```python
from build123d import *

# Parameters (mm, degrees)
SKETCH_1_R          = 16.5
EXTRUDE_1_DEPTH     = 22
SKETCH_2_R          = 18.5
EXTRUDE_2_DEPTH     = 22
SKETCH_3_R          = 6
EXTRUDE_3_DEPTH     = 6
SKETCH_4_R          = 3
EXTRUDE_7_DEPTH     = 15.5
CUT_EXTRUDE_1_DEPTH = 4
SKETCH_6_R          = 4
EXTRUDE_5_DEPTH     = 3
SKETCH_7_R          = 1.5
CUT_EXTRUDE_2_DEPTH = 6
SKETCH_8_W          = 3
SKETCH_8_H          = 0.5
EXTRUDE_6_DEPTH     = 7
SKETCH_9_W          = 2
SKETCH_9_H          = 3
CUT_EXTRUDE_3_DEPTH = 1
SKETCH_10_W         = 2
SKETCH_10_H         = 3
CUT_EXTRUDE_4_DEPTH = 1


with BuildPart() as part:
    # 草图1 → 凸台-拉伸1 (new body)
    with BuildSketch(Plane(origin=(0, 0, 0), x_dir=(1, 0, 0), z_dir=(0, 1, 0))):
        with Locations(Location((0, 0, 0), (0, 0, 270))):
            Circle(SKETCH_1_R)
    extrude(amount=EXTRUDE_1_DEPTH)

    # 草图2 → 凸台-拉伸2 (add)
    with BuildSketch(Plane(origin=(0, 22, 0), x_dir=(1, 0, 0), z_dir=(0, 1, 0))):
        with Locations(Location((0, 0, 0), (0, 0, 270))):
            Circle(SKETCH_2_R)
    extrude(amount=EXTRUDE_2_DEPTH)

    # 草图3 → 凸台-拉伸3 (add)
    with BuildSketch(Plane(origin=(0, 44, 0), x_dir=(1, 0, 0), z_dir=(0, 1, 0))):
        with Locations(Location((0, 7, 0), (0, 0, 270))):
            Circle(SKETCH_3_R)
    extrude(amount=EXTRUDE_3_DEPTH)

    # 草图4 → 凸台-拉伸7 (add)
    with BuildSketch(Plane(origin=(0, 50, 0), x_dir=(1, 0, 0), z_dir=(0, 1, 0))):
        with Locations(Location((0, 7, 0), (0, 0, 270))):
            Circle(SKETCH_4_R)
    extrude(amount=EXTRUDE_7_DEPTH)

    # 草图5 → 切除-拉伸1 (cut)
    with BuildSketch(Plane.XZ):
        with BuildLine():
            Line((-10.960155108, 8.131727984), (-8.131727984, 10.960155108))
            Line((-8.131727984, 10.960155108), (-10.16702126, 12.995448384))
            ThreePointArc((-10.16702126, 12.995448384), (-11.66726189, 11.66726189), (-12.995448384, 10.16702126))
            Line((-12.995448384, 10.16702126), (-10.960155108, 8.131727984))
        make_face()
        with BuildLine():
            Line((8.131727984, 10.960155108), (10.960155108, 8.131727984))
            Line((10.960155108, 8.131727984), (12.995448384, 10.16702126))
            ThreePointArc((12.995448384, 10.16702126), (11.66726189, 11.66726189), (10.16702126, 12.995448384))
            Line((10.16702126, 12.995448384), (8.131727984, 10.960155108))
        make_face()
        with BuildLine():
            Line((10.960155108, -8.131727984), (8.131727984, -10.960155108))
            Line((8.131727984, -10.960155108), (10.16702126, -12.995448384))
            ThreePointArc((10.16702126, -12.995448384), (11.66726189, -11.66726189), (12.995448384, -10.16702126))
            Line((12.995448384, -10.16702126), (10.960155108, -8.131727984))
        make_face()
        with BuildLine():
            Line((-8.131727984, -10.960155108), (-10.960155108, -8.131727984))
            Line((-10.960155108, -8.131727984), (-12.995448384, -10.16702126))
            ThreePointArc((-12.995448384, -10.16702126), (-11.66726189, -11.66726189), (-10.16702126, -12.995448384))
            Line((-10.16702126, -12.995448384), (-8.131727984, -10.960155108))
        make_face()
    extrude(amount=-CUT_EXTRUDE_1_DEPTH, mode=Mode.SUBTRACT)

    # 草图6 → 凸台-拉伸5 (add)
    with BuildSketch(Plane.XZ):
        with Locations(Location((0, 0, 0), (0, 0, 90))):
            Circle(SKETCH_6_R)
    extrude(amount=EXTRUDE_5_DEPTH)

    # 草图7 → 切除-拉伸2 (cut)
    with BuildSketch(Plane(origin=(0, 44, 0), x_dir=(1, 0, 0), z_dir=(0, 1, 0))):
        with Locations(Location((15.5, 0, 0), (0, 0, 270))):
            Circle(SKETCH_7_R)
        with Locations(Location((7.75, -13.423393759, 0), (0, 0, 270))):
            Circle(SKETCH_7_R)
        with Locations(Location((-7.75, -13.423393759, 0), (0, 0, 270))):
            Circle(SKETCH_7_R)
        with Locations(Location((-15.5, 0, 0), (0, 0, 270))):
            Circle(SKETCH_7_R)
        with Locations(Location((-7.75, 13.423393759, 0), (0, 0, 270))):
            Circle(SKETCH_7_R)
        with Locations(Location((7.75, 13.423393759, 0), (0, 0, 270))):
            Circle(SKETCH_7_R)
    extrude(amount=-CUT_EXTRUDE_2_DEPTH, mode=Mode.SUBTRACT)

    # 草图8 → 凸台-拉伸6 (add)
    with BuildSketch(Plane.XZ):
        with Locations((0, 11.210155108)):
            Rectangle(SKETCH_8_W, SKETCH_8_H)
        with Locations((0, -11.210155108)):
            Rectangle(SKETCH_8_W, SKETCH_8_H)
    extrude(amount=EXTRUDE_6_DEPTH)

    # 草图9 → 切除-拉伸3 (cut)
    with BuildSketch(Plane.XY.offset(11.460155108)):
        Polygon((1.5, -7), (1, -7), (1.5, -6.5), align=None)
        Polygon((-1.5, -7), (-1, -7), (-1.5, -6.5), align=None)
        with Locations((0, -4.5)):
            Rectangle(SKETCH_9_W, SKETCH_9_H)
    extrude(amount=-CUT_EXTRUDE_3_DEPTH, mode=Mode.SUBTRACT)

    # 草图10 → 切除-拉伸4 (cut)
    with BuildSketch(Plane(origin=(0, 0, -11.460155108), x_dir=(-1, 0, 0), z_dir=(0, 0, -1))):
        Polygon((1.5, -7), (1, -7), (1.5, -6.5), align=None)
        Polygon((-1.5, -7), (-1, -7), (-1.5, -6.5), align=None)
        with Locations((0, -4.5)):
            Rectangle(SKETCH_10_W, SKETCH_10_H)
    extrude(amount=-CUT_EXTRUDE_4_DEPTH, mode=Mode.SUBTRACT)


solid = part.part
```
Geometry check sheet. Reference: the model listing, model coordinates, mm. A direction names the side the tool comes from. Give positions to 0.01 mm unless a question says otherwise; leave off trailing zeros. Loops run counter-clockwise (first coordinate to the right, second up) from the corner with the lowest first, then second, coordinate; pieces in that order, holes last. Notation, with made-up numbers: M 76.5,-26 L 133.5,-26 A23 ccw 133.5,11 Z; hole C 30,18.25 d4. An arc over 180 degrees is marked long. Write item = value, one per line. Start each with the question number.
1. Section check D-D, the plane y = 45.5. Enter the section's corners in (x, z).
2. Section check B-B, the plane y = 5. Enter the section's corners in (x, z), plus the area to 3 significant figures.
3. Go/stop test with flat-tipped pins: P1, Ø1, axis at x = 14, y = 45.5, coming from the -Z side; P2, Ø12, axis at y = 48, z = 3.5, coming from the +X side; P3, Ø10, axis at y = 32.5, z = -11, coming from the +X side; P4, Ø3.5, axis at x = 0.5, y = -4, coming from the +Z side. Record where each tip stops, or that it passes through.
4. Thickness scan on probe 1 along Z at (x, y) = (7, 40); probe 2 along Y at (x, z) = (12.5, 2.5); probe 3 along Y at (x, z) = (-7.5, -14). Record the ranges inside material, lowest first.
5. Draft check along Z on faces 6 (the face through (0, -2.7, 11.46)), 7 (the face through (-11, 4, -11)), 8 (the face through (0, 44, 0)). Enter one of: +Z half, -Z half, draft (parallel to the pull), parting line (faces both ways), or undercut.
6. Tool access check on faces 1 (the face through (-11, 4, 11)), 2 (the face through (8, 38, -13)), 3 (the face through (0, 65.5, -7)), 4 (the face through (0, -2.7, -11.46)), 5 (the face through (-7.086, 32.846, 17.089)). Record the directions out of +Z, -Z, +X, -X, +Y, -Y that give a thin tool (end or side, any length) a straight path to the whole face; none if there is none.
7. Section check C-C, the plane x = 15.5. Enter the section's corners in (y, z), plus the area to 3 significant figures.
8. Section check A-A, the plane z = 0. Enter the section's corners in (x, y), plus the area to 3 significant figures.
Values follow:
q1.outline = C 0,-7 d12
q2.outline = C 0,0 d33
q2.area = 855 mm^2
q3.P1 = through
q3.P2 = 18.5
q3.P3 = 17.5
q3.P4 = 11.46
q4.probe_1 = -17.12 to -14.72, -12.12 to 12.12, 14.72 to 17.12
q4.probe_2 = 0 to 44
q4.probe_3 = 0 to 38
q5.face_6 = +Z half
q5.face_7 = undercut
q5.face_8 = draft
q6.face_1 = -Y
q6.face_2 = +Y
q6.face_3 = +Z, -Z, +X, -X, +Y
q6.face_4 = -Z, +X, -X, -Y
q6.face_5 = +Y, -Y
q7.outline = M 0,-5.66 L 22,-5.66 L 22,-10.1 L 44,-10.1 L 44,-1.5 L 38,-1.5 L 38,1.5 L 44,1.5 L 44,10.1 L 22,10.1 L 22,5.66 L 0,5.66 Z
q7.area = 675 mm^2
q8.outline = M -18.5,22 L -16.5,22 L -16.5,0 L -4,0 L -4,-3 L 4,-3 L 4,0 L 16.5,0 L 16.5,22 L 18.5,22 L 18.5,44 L 17,44 L 17,38 L 14,38 L 14,44 L -14,44 L -14,38 L -17,38 L -17,44 L -18.5,44 Z
q8.area = 1,530 mm^2
